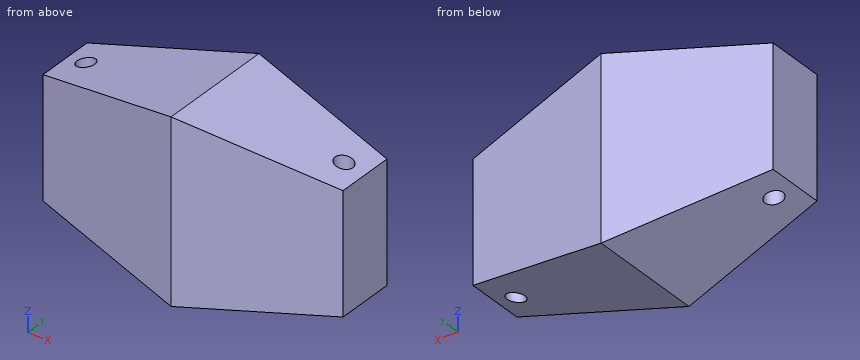
from build123d import *

# Parameters (mm, degrees)
SKETCH1_W           = 100
SKETCH1_H           = 40
BOSS_EXTRUDE1_DEPTH = 60
CUT_EXTRUDE1_DEPTH  = 40
CUT_EXTRUDE2_DEPTH  = 81.622577483
SKETCH5_R           = 3
CUT_EXTRUDE3_DEPTH  = 81.622577483


with BuildPart() as part:
    # Sketch1 → Boss-Extrude1 (new body)
    with BuildSketch(Plane.XY):
        Rectangle(SKETCH1_W, SKETCH1_H)
    extrude(amount=BOSS_EXTRUDE1_DEPTH)

    # Sketch2 → Cut-Extrude1 (cut)
    with BuildSketch(Plane(origin=(0, 20, 0), x_dir=(1, 0, 0), z_dir=(0, 1, 0))):
        Polygon((0, -60), (-50, -50), (-50, -60), align=None)
        Polygon((50, -50), (0, -60), (50, -60), align=None)
        Polygon((50, 0), (0, 0), (50, -10), align=None)
        Polygon((-50, 0), (-50, -10), (0, 0), align=None)
    extrude(amount=-CUT_EXTRUDE1_DEPTH, mode=Mode.SUBTRACT)

    # Sketch4 → Cut-Extrude2 (cut, through all)
    with BuildSketch(Plane.XY):
        Polygon((-50, 20), (0, 20), (-50, 10), align=None)
        Polygon((50, 20), (50, 10), (0, 20), align=None)
        Polygon((50, -20), (0, -20), (50, -10), align=None)
        Polygon((-50, -10), (-50, -20), (0, -20), align=None)
    extrude(amount=CUT_EXTRUDE2_DEPTH, mode=Mode.SUBTRACT)

    # Sketch5 → Cut-Extrude3 (cut, through all)
    with BuildSketch(Plane.XY):
        with Locations(Location((-43, 0, 0), (0, 0, 180))):
            Circle(SKETCH5_R)
        with Locations(Location((43, 0, 0), (0, 0, 180))):
            Circle(SKETCH5_R)
    extrude(amount=CUT_EXTRUDE3_DEPTH, mode=Mode.SUBTRACT)


solid = part.part
The model under review builds one solid part; all positions refer to its coordinate system, in mm. Coordinates: 2 decimals unless noted, no trailing zeros. Loops run counter-clockwise (first coordinate to the right, second up) from the corner with the lowest first, then second, coordinate; pieces in that order, holes last. Notation, with made-up numbers: (25, 71.5) -> (35, 71.5) arc R23 cw to (35, 104.5) -> close; hole circle Ø5 at (2.5, 82). An arc over 180 degrees is marked (long way). Use a Markdown table: item, result. Add a question column.
1. Add section B-B on z = 19. Write out the cut boundary in (x, y).
2. To check wall thickness, follow line 1 (X direction, y = 2.5, z = 45); line 2 (Y direction, x = 41, z = 51); line 3 (Y direction, x = -43, z = 38). State the ranges of each line that lie inside material, in increasing order.
3. Clearance check with flat-ended pins moving along their axes: pin 1 Ø7 at (x, y) = (-43, 0) entering from -Z; pin 2 Ø6 at (x, z) = (-25, 38) entering from +Y; pin 3 Ø4 at (x, z) = (10, 39.5) entering from -Y. State where each tip first meets the part, or that it passes through.
4. Add section D-D on y = 11.5. Write out the cut boundary in (x, z).
5. Add section C-C on x = -43. Write out the cut boundary in (y, z).
6. Add section A-A on y = 0. Write out the cut boundary in (x, z).
Returned:
| question | item | result |
|---|---|---|
| 1 | outline | (-50, -10) -> (0, -20) -> (50, -10) -> (50, 10) -> (0, 20) -> (-50, 10) -> close; hole circle Ø6 at (-43, 0); hole circle Ø6 at (43, 0) |
| 2 | line 1 | x = -50 to -44.66, -41.34 to 41.34, 44.66 to 50 |
| 2 | line 2 | y = -11.8 to -2.24, 2.24 to 11.8 |
| 2 | line 3 | y = -11.4 to -3, 3 to 11.4 |
| 3 | pin 1 | stops at z = 7.9 |
| 3 | pin 2 | stops at y = 15.6 |
| 3 | pin 3 | stops at y = -18.4 |
| 4 | outline | (-42.5, 8.5) -> (0, 0) -> (42.5, 8.5) -> (42.5, 51.5) -> (0, 60) -> (-42.5, 51.5) -> close |
| 5 | outline | (-11.4, 8.6) -> (-3, 8.6) -> (-3, 51.4) -> (-11.4, 51.4) -> close; (3, 8.6) -> (11.4, 8.6) -> (11.4, 51.4) -> (3, 51.4) -> close |
| 6 | outline | (-50, 10) -> (-46, 9.2) -> (-46, 50.8) -> (-50, 50) -> close; (-40, 8) -> (0, 0) -> (40, 8) -> (40, 52) -> (0, 60) -> (-40, 52) -> close; (46, 9.2) -> (50, 10) -> (50, 50) -> (46, 50.8) -> close |
